```python
from build123d import *

# Parameters (mm, degrees)
SKETCH1_W          = 60
SKETCH1_H          = 60
BASE_FLANGE1_DEPTH = 3
EDGE_FLANGE1_DEPTH = 60
EDGE_FLANGE2_DEPTH = 60
FILLET1_R          = 10
SKETCH12_R         = 2.55
CUT_EXTRUDE1_DEPTH = 10
CAVITY1_START      = -1.5
CAVITY1_DEPTH      = 3
SKETCH15_W         = 15.4
SKETCH15_H         = 3.400000894
SKETCH15_H_2       = 3.4
CUT_EXTRUDE3_DEPTH = 3
SKETCH16_R         = 1.5
CUT_EXTRUDE4_DEPTH = 3
SKETCH17_R         = 2.55
CUT_EXTRUDE5_DEPTH = 10


# Read off the part's stored shape, not the designer's step: Cavity1
# Sheet-metal steps are written as plain solids
with BuildPart() as part:
    # Sketch1 → Base-Flange1 (new body)
    with BuildSketch(Plane(origin=(0, 0, 0), x_dir=(1, 0, 0), z_dir=(0, 1, 0))):
        Rectangle(SKETCH1_W, SKETCH1_H)
    extrude(amount=-BASE_FLANGE1_DEPTH)

    # Edge-Flange1 section (across the edge) → Edge-Flange1 (add)
    with BuildSketch(Plane(origin=(30.705307923, 0, 30), x_dir=(-0.3420201433256631, 0.9396926207859105, 0), z_dir=(0, 0, -1))):
        with BuildLine():
            Line((-3, 0.705307923), (-3, 199.471019058))
            Line((-3, 199.471019058), (0, 199.471019058))
            Line((0, 199.471019058), (0, 0.705307923))
            ThreePointArc((0, 0.705307923), (0.060768988, 0.010715212), (0.241229517, -0.66277265))
            Line((0.241229517, -0.66277265), (-2.577848346, -1.68883308))
            ThreePointArc((-2.577848346, -1.68883308), (-2.893654271, -0.510229321), (-3, 0.705307923))
        make_face()
    extrude(amount=EDGE_FLANGE1_DEPTH)

    # Edge-Flange2 section (across the edge) → Edge-Flange2 (add)
    with BuildSketch(Plane(origin=(219.835585673, 65.645258182, -30), x_dir=(0, -1, 0), z_dir=(0, 0, 1))):
        with BuildLine():
            Line((-3, 0.705307923), (-3, 79.471019058))
            Line((-3, 79.471019058), (0, 79.471019058))
            Line((0, 79.471019058), (0, 0.705307923))
            ThreePointArc((0, 0.705307923), (0.060768988, 0.010715212), (0.241229517, -0.66277265))
            Line((0.241229517, -0.66277265), (-2.577848346, -1.68883308))
            ThreePointArc((-2.577848346, -1.68883308), (-2.893654271, -0.510229321), (-3, 0.705307923))
        make_face()
    extrude(amount=EDGE_FLANGE2_DEPTH)

    # Fillet1
    fillet1_edges = [part.edges().sort_by_distance(p)[0] for p in [
        (299.30660473, 67.145258182, -30),
        (299.30660473, 67.145258182, 30),
        (-30, -1.5, 30),
        (-30, -1.5, -30),
    ]]
    fillet(fillet1_edges, radius=FILLET1_R)

    # Sketch12 → Cut-Extrude1 (cut)
    with BuildSketch(Plane(origin=(0, 0, 0), x_dir=(1, 0, 0), z_dir=(0, 1, 0))):
        with Locations(Location((20, 20, 0), (0, 0, 270))):
            Circle(SKETCH12_R)
        with Locations(Location((20, -20, 0), (0, 0, 270))):
            Circle(SKETCH12_R)
        with Locations(Location((-20, -20, 0), (0, 0, 270))):
            Circle(SKETCH12_R)
        with Locations(Location((-20, 20, 0), (0, 0, 270))):
            Circle(SKETCH12_R)
        with Locations(Location((-20, 0, 0), (0, 0, 270))):
            Circle(SKETCH12_R)
        with Locations(Location((20, 0, 0), (0, 0, 270))):
            Circle(SKETCH12_R)
    extrude(amount=-CUT_EXTRUDE1_DEPTH, mode=Mode.SUBTRACT)

    # Cavity1 outline → Cavity1 (cut)
    with BuildSketch(Plane.XY.offset(CAVITY1_START)):
        with BuildLine():
            ThreePointArc((167.585662257, 46.627841316), (168.714237544, 47.661990034), (168.781007212, 49.191266844))
            Line((168.781007212, 49.191266844), (168.438987069, 50.130959465))
            Line((168.438987069, 50.130959465), (154.343597757, 45.000657315))
            Line((154.343597757, 45.000657315), (154.6856179, 44.060964694))
            ThreePointArc((154.6856179, 44.060964694), (155.719766618, 42.932389407), (157.249043428, 42.865619739))
            Line((157.249043428, 42.865619739), (167.585662257, 46.627841316))
        make_face()
        with BuildLine():
            Line((109.317258169, 27.548232175), (108.975238025, 28.487924795))
            Line((108.975238025, 28.487924795), (94.879848713, 23.357622645))
            Line((94.879848713, 23.357622645), (95.221868857, 22.417930025))
            ThreePointArc((95.221868857, 22.417930025), (96.256017575, 21.289354737), (97.785294385, 21.22258507))
            Line((97.785294385, 21.22258507), (108.121913214, 24.984806646))
            ThreePointArc((108.121913214, 24.984806646), (109.250488501, 26.018955365), (109.317258169, 27.548232175))
        make_face()
        with BuildLine():
            Line((59.726286316, 9.498594532), (59.384266173, 10.438287153))
            Line((59.384266173, 10.438287153), (45.288876861, 5.307985003))
            Line((45.288876861, 5.307985003), (45.630897004, 4.368292382))
            ThreePointArc((45.630897004, 4.368292382), (46.665045723, 3.239717095), (48.194322533, 3.172947427))
            Line((48.194322533, 3.172947427), (58.530941361, 6.935169004))
            ThreePointArc((58.530941361, 6.935169004), (59.659516649, 7.969317722), (59.726286316, 9.498594532))
        make_face()
    extrude(amount=CAVITY1_DEPTH, mode=Mode.SUBTRACT)

    # Sketch15 → Cut-Extrude3 (cut)
    with BuildSketch(Plane(origin=(3.591838707, -9.868495742, 0), x_dir=(0.9396926207859104, 0.34202014332566316, 0), z_dir=(-0.34202014332566316, 0.9396926207859104, 0))):
        with Locations((104.646671142, 0)):
            Rectangle(SKETCH15_W, SKETCH15_H)
        with Locations((51.873061181, 0)):
            Rectangle(SKETCH15_W, SKETCH15_H)
        with Locations((167.926671142, 0)):
            Rectangle(SKETCH15_W, SKETCH15_H_2)
    extrude(amount=-CUT_EXTRUDE3_DEPTH, mode=Mode.SUBTRACT)

    # Sketch16 → Cut-Extrude4 (cut)
    with BuildSketch(Plane(origin=(0, 68.645258182, 0), x_dir=(1, 0, 0), z_dir=(0, 1, 0))):
        with Locations(Location((265.60660473, 0, 0), (0, 0, 270))):
            Circle(SKETCH16_R)
        with Locations(Location((241.60660473, 14.5, 0), (0, 0, 270))):
            Circle(SKETCH16_R)
        with Locations(Location((241.60660473, -14.5, 0), (0, 0, 270))):
            Circle(SKETCH16_R)
    extrude(amount=-CUT_EXTRUDE4_DEPTH, mode=Mode.SUBTRACT)

    # Sketch17 → Cut-Extrude5 (cut)
    with BuildSketch(Plane(origin=(3.591838707, -9.868495742, 0), x_dir=(0.9396926207859104, 0.34202014332566316, 0), z_dir=(-0.34202014332566316, 0.9396926207859104, 0))):
        with Locations(Location((136.324570332, 0, 0), (0, 0, 180))):
            Circle(SKETCH17_R)
        with Locations(Location((201.324570332, 0, 0), (0, 0, 180))):
            Circle(SKETCH17_R)
        with Locations(Location((73.074570332, 0, 0), (0, 0, 180))):
            Circle(SKETCH17_R)
    extrude(amount=-CUT_EXTRUDE5_DEPTH, mode=Mode.SUBTRACT)


solid = part.part
```
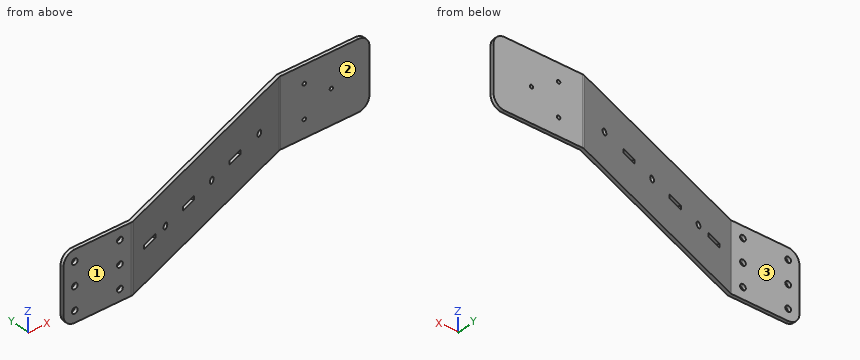
Model file for the job. Use its own axes, mm. Face numbers are marked on the shaded views. A direction names the side the tool comes from. Coordinates: 2 decimals unless noted, no trailing zeros. Order: outer loops, then holes, each group sorted by start corner. A loop starts at its lowest first (then second) coordinate and runs counter-clockwise, first axis right, second up. Notation, with made-up numbers: (11, -17.75) - (61, -17.75) arc R17 ccw to (61, 12.25) - close; hole circle Ø8 at (25, 2). An arc over 180 degrees is marked (long way). Return JSON: item names as keys, results as strings. Group by question number.
1) Saw through at B-B, the plane x = -4.5. Write the cut outline in (y, z), plus the area to 3 significant figures.
2) Saw through at A-A, the plane x = 56. Write the cut outline in (y, z), plus the area to 3 significant figures.
3) Tool access for the marked faces 1, 2 and 3: list every direction of +Z, -Z, +X, -X, +Y, -Y with a clear straight run to the whole face (end or side of a thin tool).
4) Saw through at C-C, the plane x = 118. Write the cut outline in (y, z).
5) Probe line 1 (Y direction, x = 275.5, z = -19); line 2 (Y direction, x = 4.5, z = -12). List the from-to ranges inside material, lowest first. Write a range as from..to.
6) Flat gauge pins, fed straight in: P1, Ø12, axis at x = 214.5, z = 15.5, coming from the -Y side; P2, Ø6.5, axis at x = 20, z = -20, coming from the +Y side; P3, Ø3, axis at x = -20, z = 0, coming from the +Y side; P4, Ø6, axis at x = 68.5, z = -6.5, coming from the +Y side. Where does each tip first touch, or does it go through?
Values found:
{
 "1": {"outline": "(-3, -30) - (0, -30) - (0, 30) - (-3, 30) - close", "area": "180 mm²"},
 "2": {"outline": "(6.01, -30) - (9.21, -30) - (9.21, -1.7) - (6.01, -1.7) - close; (6.01, 1.7) - (9.21, 1.7) - (9.21, 30) - (6.01, 30) - close", "area": "181 mm²"},
 "3": {"face 1": "+Z, -Z, +X, -X, -Y", "face 2": "+Z, -Z, +X, -Y", "face 3": "+Z, -Z, -X, +Y"},
 "4": {"outline": "(28.58, -30) - (31.77, -30) - (31.77, 30) - (28.58, 30) - close"},
 "5": {"line 1": "y = 65.65..68.65", "line 2": "y = -3..0"},
 "6": {"P1": "stops at y = 61.52", "P2": "stops at y = 0", "P3": "passes through", "P4": "stops at y = 14.85"}
}
